Could you check a few things on this model? Use its own coordinates, in mm. Face numbers are marked on the shaded views. A direction names the side the tool comes from. Give positions to 0.01 mm unless a question says otherwise; leave off trailing zeros. Order: outer loops, then holes, each group sorted by start corner. A loop starts at its lowest first (then second) coordinate and runs counter-clockwise, first axis right, second up. Notation, with made-up numbers: M 54,-29.5 L 91,-29.5 A22 ccw 91,-21.5 Z; hole C 53,87.25 d6. An arc over 180 degrees is marked long. Use a Markdown table: item, result. Add a question column.
Item 1: Suppose I cut it at C-C on x = 20. Write out the boundary of the cut face in (y, z).
Item 2: If I drill on L1, parallel to Y at x = 7, z = 0; L2, parallel to X at y = -9, z = -20; L3, parallel to X at y = -4.5, z = 13, over which ranges is the centre line in solid material (lowest first)? Write a range as from..to.
Item 3: Suppose I cut it at A-A on z = 0. Count the separate pieces of the cut face and the enclosed holes in it, plus the area to 3 significant figures.
Item 4: I'm going to push flat-ended pins straight in: pin 1 Ø12 at (x, y) = (9.5, 10) entering from -Z; pin 2 Ø5 at (y, z) = (7.5, -6.5) entering from -X; pin 3 Ø6 at (x, y) = (30, 12) entering from +Z; pin 4 Ø5 at (y, z) = (0, 19.84) entering from -X. Where does each tip first touch, or does it pass through?
Item 5: For the marked faces 1, 2 and 3, which set-ups out of +Z, -Z, +X, -X, +Y, -Y let a thin tool reach every point of the face, with its end or its side?
from build123d import *

# Parameters (mm, degrees)
FILLET1_R          = 2.3876
CHAMFER1_SIZE      = 0.762
CHAMFER2_SIZE      = 1.524
CUT_EXTRUDE2_START = 14.351
SKETCH2_R          = 2.7686
CUT_EXTRUDE2_DEPTH = 76.325619122
CUT_EXTRUDE4_START = 14.351
SKETCH3_R          = 2.7686
CUT_EXTRUDE4_DEPTH = 76.325619122


with BuildPart() as part:
    # Sketch1 → Revolve1 (revolve)
    with BuildSketch(Plane(origin=(0, 0, 0), x_dir=(0, 1, 0), z_dir=(0, 0, 1)), mode=Mode.PRIVATE) as revolve1_sk:
        Polygon((0, 0), (8.7122, 0), (8.7122, -4.826), (24.6126, -4.826), (24.6126, -14.351), (12.7, -14.351), (12.7, -50.0634), (0, -50.0634), align=None)
    revolve(revolve1_sk.sketch.rotate(Axis((-25.4, 0, 0), (1, 0, 0)), 90), axis=Axis((-25.4, 0, 0), (1, 0, 0)))

    # Fillet1
    fillet1_edges = [part.edges().sort_by_distance(p)[0] for p in [
        (14.351, 0, -12.7),
    ]]
    fillet(fillet1_edges, radius=FILLET1_R)

    # Chamfer1
    chamfer1_edges = [part.edges().sort_by_distance(p)[0] for p in [
        (14.351, 0, -24.6126),
        (4.826, 0, -24.6126),
        (0, 0, -8.7122),
    ]]
    chamfer(chamfer1_edges, length=CHAMFER1_SIZE)

    # Chamfer2
    chamfer2_edges = [part.edges().sort_by_distance(p)[0] for p in [
        (50.0634, 0, -12.7),
    ]]
    chamfer(chamfer2_edges, length=CHAMFER2_SIZE)

    # Sketch2 → Cut-Extrude2 (cut, through all)
    with BuildSketch(Plane.YZ.offset(CUT_EXTRUDE2_START)):
        with Locations(Location((19.8374, 0, 0), (0, 0, 270))):
            Circle(SKETCH2_R)
    extrude(amount=-CUT_EXTRUDE2_DEPTH, mode=Mode.SUBTRACT)

    # Sketch3 → Cut-Extrude4 (cut, through all)
    with BuildSketch(Plane.YZ.offset(CUT_EXTRUDE4_START)):
        with Locations(Location((0, 19.8374, 0), (0, 0, 270))):
            Circle(SKETCH3_R)
        with Locations(Location((-19.8374, 0, 0), (0, 0, 270))):
            Circle(SKETCH3_R)
        with Locations(Location((0, -19.8374, 0), (0, 0, 270))):
            Circle(SKETCH3_R)
    extrude(amount=-CUT_EXTRUDE4_DEPTH, mode=Mode.SUBTRACT)


solid = part.part
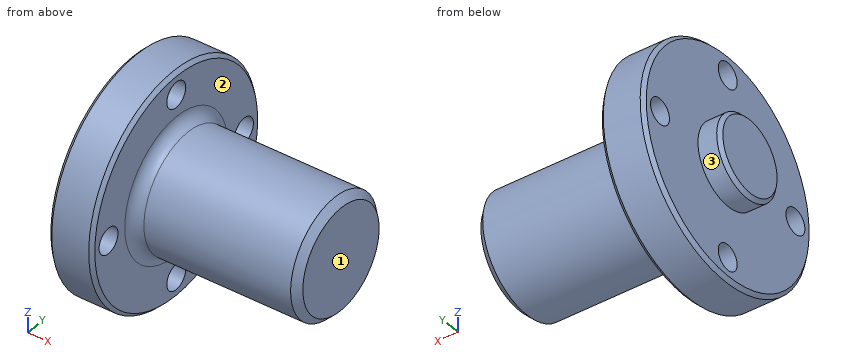
Findings below:
| question | item | result |
|---|---|---|
| 1 | outline | C 0,0 d25.4 |
| 2 | L1 | y = -24.61..-22.61, -17.07..17.07, 22.61..24.61 |
| 2 | L2 | x = 4.83..14.35 |
| 2 | L3 | x = 4.83..14.76 |
| 3 | separate pieces | 3 |
| 3 | enclosed holes | 0 |
| 3 | area | 1,350 mm^2 |
| 4 | pin 1 | stops at z = -24.29 |
| 4 | pin 2 | stops at x = 0 |
| 4 | pin 3 | stops at z = 8.96 |
| 4 | pin 4 | passes through |
| 5 | face 1 | +Z, -Z, +X, +Y, -Y |
| 5 | face 2 | +X |
| 5 | face 3 | -X |
